from build123d import *

# Parameters (mm, degrees)
BOSS_EXTRUDE1_DEPTH      = 100
CUT_EXTRUDE1_START       = -5
SKETCH2_R                = 41
CUT_EXTRUDE1_DEPTH       = 184.085087128
SKETCH3_R                = 15
CUT_EXTRUDE2_DEPTH       = 10
CUT_EXTRUDE3_DEPTH       = 187.732428892
CUT_EXTRUDE3_DEPTH_BACK  = 187.732428892
SKETCH4_R                = 3
M4_CLEARANCE_HOLE2_D     = 4.8
M4_CLEARANCE_HOLE2_DEPTH = 5
M4_CLEARANCE_HOLE2_TIP   = 1.442065486
SKETCH10_R               = 26
CUT_EXTRUDE5_DEPTH       = 193
M6_CLEARANCE_HOLE1_D     = 6.4
CUT_EXTRUDE6_START       = -1
SKETCH14_R               = 27.6
CUT_EXTRUDE6_DEPTH       = 1
CUT_EXTRUDE7_START       = -9
SKETCH14_2_R             = 27.6
CUT_EXTRUDE7_DEPTH       = 1
CUT_EXTRUDE8_START       = -2
SKETCH15_R               = 27.6
CUT_EXTRUDE8_DEPTH       = 1
CUT_EXTRUDE9_START       = -10
SKETCH15_2_R             = 27.6
CUT_EXTRUDE9_DEPTH       = 1


with BuildPart() as part:
    # Sketch1 → Boss-Extrude1 (new body)
    with BuildSketch(Plane.XY):
        Polygon((0, 0), (0, 110), (11, 110), (11, 10), (113, 10), (113, 110), (124, 110), (124, 0), align=None)
    extrude(amount=BOSS_EXTRUDE1_DEPTH)

    # Sketch2 → Cut-Extrude1 (cut, through all)
    with BuildSketch(Plane(origin=(0, 10, 0), x_dir=(1, 0, 0), z_dir=(0, 1, 0)).offset(CUT_EXTRUDE1_START)):
        with Locations(Location((62, -50, 0), (0, 0, 270))):
            Circle(SKETCH2_R)
    extrude(amount=-CUT_EXTRUDE1_DEPTH, mode=Mode.SUBTRACT)

    # Sketch3 → Cut-Extrude2 (cut)
    with BuildSketch(Plane.XZ.offset(-5)):
        with Locations(Location((62, 50, 0), (0, 0, 270))):
            Circle(SKETCH3_R)
    extrude(amount=-CUT_EXTRUDE2_DEPTH, mode=Mode.SUBTRACT)

    # Sketch4 → Cut-Extrude3 (cut, two sides: drawn at the far end of the back side and taken through both)
    with BuildSketch(Plane(origin=(11, 0, 0), x_dir=(0, 0, -1), z_dir=(1, 0, 0)).offset(-CUT_EXTRUDE3_DEPTH_BACK)):
        with Locations(Location((-9.341360082, 19.341360082, 0), (0, 0, 90))):
            Circle(SKETCH4_R)
        with Locations(Location((-90.658639918, 19.341360082, 0), (0, 0, 90))):
            Circle(SKETCH4_R)
        with Locations(Location((-90.658639918, 100.658639918, 0), (0, 0, 90))):
            Circle(SKETCH4_R)
        with Locations(Location((-9.341360082, 100.658639918, 0), (0, 0, 90))):
            Circle(SKETCH4_R)
        with Locations((7.5, 60)):
            Circle(SKETCH4_R)
    extrude(amount=CUT_EXTRUDE3_DEPTH + CUT_EXTRUDE3_DEPTH_BACK, mode=Mode.SUBTRACT)

    # M4 Clearance Hole2
    with Locations(Plane(origin=(0, 10, 0), x_dir=(1, 0, 0), z_dir=(0, 1, 0))):
        with Locations((69.403965408, -30.348503969), (91, -50), (71.348503969, -71.596034592), (49.752469377, -51.944538562)):
            Hole(M4_CLEARANCE_HOLE2_D / 2, depth=M4_CLEARANCE_HOLE2_DEPTH)
            with Locations((0, 0, -(M4_CLEARANCE_HOLE2_DEPTH + M4_CLEARANCE_HOLE2_TIP / 2))):  # 118° drill point
                Cone(0, M4_CLEARANCE_HOLE2_D / 2, M4_CLEARANCE_HOLE2_TIP, mode=Mode.SUBTRACT)

    # Sketch10 → Cut-Extrude5 (cut)
    with BuildSketch(Plane(origin=(124, 0, 0), x_dir=(0, 0, -1), z_dir=(1, 0, 0))):
        with Locations((-50, 60)):
            Circle(SKETCH10_R)
    extrude(amount=-CUT_EXTRUDE5_DEPTH, mode=Mode.SUBTRACT)

    # M6 Clearance Hole1 (through all)
    with Locations(Plane(origin=(124, 0, 0), x_dir=(0, 0, -1), z_dir=(1, 0, 0))):
        with Locations((-72.980970389, 82.980970389), (-50, 92.5), (-27.019029611, 82.980970389), (-17.5, 60), (-27.019029611, 37.019029611), (-50, 27.5), (-72.980970389, 37.019029611), (-82.5, 60)):
            Hole(M6_CLEARANCE_HOLE1_D / 2)

    # Sketch14 → Cut-Extrude6 (cut)
    with BuildSketch(Plane(origin=(124, 0, 0), x_dir=(0, 0, -1), z_dir=(1, 0, 0)).offset(CUT_EXTRUDE6_START)):
        with Locations(Location((-50, 60, 0), (0, 0, 90))):
            Circle(SKETCH14_R)
    extrude(amount=-CUT_EXTRUDE6_DEPTH, mode=Mode.SUBTRACT)

    # Sketch14_2 → Cut-Extrude7 (cut)
    with BuildSketch(Plane(origin=(124, 0, 0), x_dir=(0, 0, -1), z_dir=(1, 0, 0)).offset(CUT_EXTRUDE7_START)):
        with Locations(Location((-50, 60, 0), (0, 0, 90))):
            Circle(SKETCH14_2_R)
    extrude(amount=-CUT_EXTRUDE7_DEPTH, mode=Mode.SUBTRACT)

    # Sketch15 → Cut-Extrude8 (cut)
    with BuildSketch(Plane.ZY.offset(CUT_EXTRUDE8_START)):
        with Locations(Location((50, 60, 0), (0, 0, 90))):
            Circle(SKETCH15_R)
    extrude(amount=CUT_EXTRUDE8_DEPTH, mode=Mode.SUBTRACT)

    # Sketch15_2 → Cut-Extrude9 (cut)
    with BuildSketch(Plane.ZY.offset(CUT_EXTRUDE9_START)):
        with Locations(Location((50, 60, 0), (0, 0, 90))):
            Circle(SKETCH15_2_R)
    extrude(amount=CUT_EXTRUDE9_DEPTH, mode=Mode.SUBTRACT)


solid = part.part
Verification items for the finished model (mm, model axes). A direction names the side the tool comes from. Give positions to 0.01 mm unless a question says otherwise; leave off trailing zeros. Loops run counter-clockwise (first coordinate to the right, second up) from the corner with the lowest first, then second, coordinate; pieces in that order, holes last.
1. Cross-section at C-C on z = 82.5. Record the cut outline in (x, y) (3 decimals).
Derived:
outline: (0, 0) - (37.005, 0) - (37.005, 5) - (86.995, 5) - (86.995, 0) - (124, 0) - (124, 56.8) - (113, 56.8) - (113, 10) - (11, 10) - (11, 56.8) - (0, 56.8) - close; (0, 63.2) - (11, 63.2) - (11, 110) - (0, 110) - close; (113, 63.2) - (124, 63.2) - (124, 110) - (113, 110) - close
2. Cross-section at A-A on x = 62. Record the cut outline in (y, z), and give its area (3 significant figures).
Derived:
outline: (0, 0) - (10, 0) - (10, 35) - (5, 35) - (5, 9) - (0, 9) - close; (0, 91) - (5, 91) - (5, 65) - (10, 65) - (10, 100) - (0, 100) - close
area: 440 mm2
3. Go/stop test with flat-tipped pins: P1, Ø2, axis at x = 104.5, z = 64.5, coming from the +Y side; P2, Ø5, axis at x = 47, z = 29, coming from the -Y side. Record where each tip stops, or that it passes through.
Derived:
P1: stops at y = 10
P2: stops at y = 5
4. Tool access check on faces 1 (the flat face through (5, 110, 49)), 2 (the flat face through (113, 70, 83)), 3 (the cylindrical face through (9.507, 85.495, 60.571)). Record the directions out of +Z, -Z, +X, -X, +Y, -Y that give a thin tool (end or side, any length) a straight path to the whole face; none if there is none.
Derived:
face 1: +Z, -Z, +X, -X, +Y
face 2: +Z, -Z, +Y
face 3: none
5. Material ranges on probe 1 along X at (y, z) = (83, 35.5); probe 2 along Y at (x, z) = (7.5, 50); probe 3 along Z at (x, y) = (3, 27), recorded low to high.
Derived:
probe 1: x = 0 to 1, 2 to 9, 10 to 11, 113 to 114, 115 to 122, 123 to 124
probe 2: y = 0 to 24.3, 30.7 to 34, 86 to 89.3, 95.7 to 110
probe 3: z = 0 to 46.84, 53.16 to 100
6. Cross-section at D-D on z = 50. Count the separate pieces of the cut face and the enclosed holes in it, and give its area (3 significant figures).
Derived:
separate pieces: 9
enclosed holes: 0
area: 1,420 mm2
7. Release check for a two-part mould opening along X. For faces 4 (the cylindrical face through (1.507, 85.495, 60.571)), 5 (the flat face through (2, 41, 68)), 6 (the cylindrical face through (5.423, 17.13, 92.686)) record: +X half, -X half, draft (parallel to the pull), parting line (faces both ways), or undercut.
Derived:
face 4: undercut
face 5: undercut
face 6: draft
8. Cross-section at B-B on y = 92.5. Record the cut outline in (x, z).
Derived:
outline: (0, 0) - (11, 0) - (11, 46.8) - (0, 46.8) - close; (0, 53.2) - (11, 53.2) - (11, 100) - (0, 100) - close; (113, 0) - (124, 0) - (124, 46.8) - (113, 46.8) - close; (113, 53.2) - (124, 53.2) - (124, 100) - (113, 100) - close
